For this review, take the finished solid that the model builds, in its own axes (mm). Give positions to 0.01 mm unless a question says otherwise; leave off trailing zeros. Order: outer loops, then holes, each group sorted by start corner. A loop starts at its lowest first (then second) coordinate and runs counter-clockwise, first axis right, second up.
Autodesk Inventor part; units mm, degrees
ref_plane "YZ Plane" through (0, 0, 0) normal (1, 0, 0) x (0, 1, 0)
ref_plane "XZ Plane" through (0, 0, 0) normal (0, 1, 0) x (-1, 0, 0)
ref_plane "XY Plane" through (0, 0, 0) normal (0, 0, 1) x (1, 0, 0)
sketch "Sketch1" plane through (0, 0, 0) normal (0, 0, 1) x (1, 0, 0)
  line L0 (-12.7, -12.7) -> (12.7, -12.7)
  line L1 (12.7, -12.7) -> (12.7, 12.7)
  line L2 (12.7, 12.7) -> (-12.7, 12.7)
  line L3 (-12.7, 12.7) -> (-12.7, -12.7)
  line L4 (-11.1125, -11.1125) -> (11.1125, -11.1125)
  line L5 (11.1125, -11.1125) -> (11.1125, 11.1125)
  line L6 (11.1125, 11.1125) -> (-11.1125, 11.1125)
  line L7 (-11.1125, 11.1125) -> (-11.1125, -11.1125)
  point P0 (0, 0)
  dimension "d0" = 25.4
  dimension "d1" = 25.4
  dimension "d2" = 22.225
  dimension "d3" = 22.225
extrude "Extrusion1" add sketch "Sketch1" along normal blind 711.2
equation "\"BendRadius\" = Thickness"
equation "\"BendReliefWidth\" = Thickness"
equation "\"BendReliefDepth\" = 0.5 * Thickness"
equation "\"CornerReliefSize\" = 4 * Thickness"
equation "\"MinimumRemnant\" = 2 * Thickness"
equation "\"TransitionRadius\" = BendRadius"
equation "\"JacobiRadiusSize\" = BendRadius"
equation "\"GapSize\" = Thickness"
properties part number "28 in 1-16"
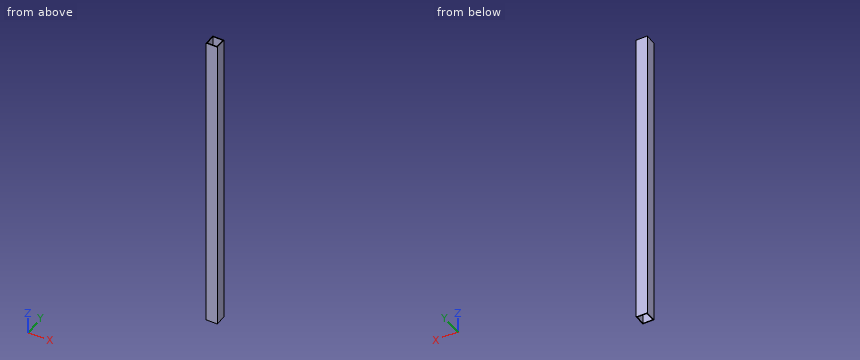
1) We need section A-A on x = 7. Give the boundary of the cut face in (y, z), then the cut area to 3 significant figures.
Answer sheet:
outline: (-12.7, 0) - (-11.11, 0) - (-11.11, 711.2) - (-12.7, 711.2) - close; (11.11, 0) - (12.7, 0) - (12.7, 711.2) - (11.11, 711.2) - close
area: 2,260 mm2
2) Clearance check with a flat-ended pin moving along its axis: pin 1 (12 mm diameter, centred on x = -4, y = -3, fed in from +Z). State where the tip first meets the part, or that it passes through.
Answer sheet:
pin 1: passes through
3) We need section B-B on z = 553.5. Give the boundary of the cut face in (x, y).
Answer sheet:
outline: (-12.7, -12.7) - (12.7, -12.7) - (12.7, 12.7) - (-12.7, 12.7) - close; hole (-11.11, -11.11) - (11.11, -11.11) - (11.11, 11.11) - (-11.11, 11.11) - close
4) To check wall thickness, follow line 1 (Y direction, x = -0.25, z = 152). State the ranges of the line that lie inside material, in increasing order.
Answer sheet:
line 1: y = -12.7 to -11.11, 11.11 to 12.7
